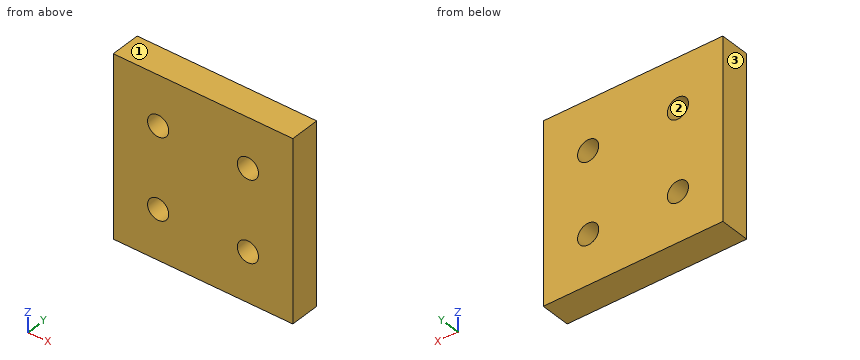
Autodesk Inventor part; units mm, degrees
ref_plane "YZ Plane" through (0, 0, 0) normal (1, 0, 0) x (0, 1, 0)
ref_plane "XZ Plane" through (0, 0, 0) normal (0, 1, 0) x (-1, 0, 0)
ref_plane "XY Plane" through (0, 0, 0) normal (0, 0, 1) x (1, 0, 0)
sketch "Sketch1" plane through (0, 0, 0) normal (0, 1, 0) x (-1, 0, 0)
  line L0 (-19.05, 19.05) -> (19.05, 19.05)
  line L1 (19.05, 19.05) -> (19.05, -19.05)
  line L2 (19.05, -19.05) -> (-19.05, -19.05)
  line L3 (-19.05, -19.05) -> (-19.05, 19.05)
  line L4 (-19.05, 19.05) -> (19.05, -19.05) construction
  line L5 (19.05, 19.05) -> (-19.05, -19.05) construction
  point P0 (0, 0)
  dimension "d0" = 38.1
  dimension "d1" = 38.1
extrude "Extrusion1" add sketch "Sketch1" along normal blind 6.35
sketch "Sketch2" plane through (0, 6.35, 0) normal (0, 1, 0) x (1, 0, 0)
  line L0 (-19.05, -19.05) -> (19.05, -19.05) construction
  line L1 (19.05, -19.05) -> (19.05, 19.05) construction
  line L2 (19.05, 19.05) -> (-19.05, 19.05) construction
  line L3 (-19.05, 19.05) -> (-19.05, -19.05) construction
  point P0 (0, 0)
  point P1 (-9.525, -8.5725)
  point P2 (-9.525, 8.5725)
  point P3 (9.525, -8.5725)
  point P4 (9.525, 8.5725)
  dimension "d6" = 17.145
  dimension "d9" = 19.05
  dimension "d12" = 8.5725
  dimension "d13" = 9.525
hole "Hole1" at (-9.525, 6.35, 8.5725) at (-9.525, 6.35, -8.5725) at (9.525, 6.35, 8.5725) at (9.525, 6.35, -8.5725) direction (0, -1, 0) diameter 4.4958 end through all
properties part number "holestandard" material "Aluminum 6061"
Part model, mm, in its own coordinate system. Face numbers are marked on the shaded views. Coordinates: 2 decimals unless noted, no trailing zeros. Order: outer loops, then holes, each group sorted by start corner. A loop starts at its lowest first (then second) coordinate and runs counter-clockwise, first axis right, second up. Notation, with made-up numbers: M 80.5,0 L 119.5,0 A17 cw 119.5,15 Z; hole C 70,-34 d3. An arc over 180 degrees is marked long. Use a Markdown table: item, result.
(1) Flat gauge pin, fed straight in: pin 1 (7 mm diameter, centred on x = 9.52, z = 8.57, fed in from +Y). Where does the tip first touch, or does it go through?
A:
| item | result |
|---|---|
| pin 1 | stops at y = 6.35 |
(2) Cut at A-A on z = 7. Write the cut outline in (x, y), then the cut area to 3 significant figures.
A:
| item | result |
|---|---|
| outline | M -19.05,0 L -11.13,0 L -11.13,6.35 L -19.05,6.35 Z; M -7.92,0 L 7.92,0 L 7.92,6.35 L -7.92,6.35 Z; M 11.13,0 L 19.05,0 L 19.05,6.35 L 11.13,6.35 Z |
| area | 201 mm^2 |
(3) Pull direction X, two halves, no side cores. Call the marked faces 1, 2 and 3: released by +X, released by -X, zero draft, split by the parting line, or undercut.
A:
| item | result |
|---|---|
| face 1 | zero draft |
| face 2 | undercut |
| face 3 | released by -X |
(4) Cut at C-C on y = 4. State how many separate pieces and enclosed holes the cut face has, then the cut area to 3 significant figures.
A:
| item | result |
|---|---|
| separate pieces | 1 |
| enclosed holes | 4 |
| area | 1,390 mm^2 |
(5) Cut at B-B on x = 10.5. Write the cut outline in (y, z).
A:
| item | result |
|---|---|
| outline | M 0,-19.05 L 6.35,-19.05 L 6.35,-10.6 L 0,-10.6 Z; M 0,-6.55 L 6.35,-6.55 L 6.35,6.55 L 0,6.55 Z; M 0,10.6 L 6.35,10.6 L 6.35,19.05 L 0,19.05 Z |
(6) Probe L1, parallel to X at y = 5.25, z = 7.5; L2, parallel to X at y = 2.75, z = 9; L3, parallel to Z at x = 8.5, y = 0.75. List the from-to ranges inside material, lowest first.
A:
| item | result |
|---|---|
| L1 | x = -19.05 to -11.5, -7.55 to 7.55, 11.5 to 19.05 |
| L2 | x = -19.05 to -11.73, -7.32 to 7.32, 11.73 to 19.05 |
| L3 | z = -19.05 to -10.57, -6.57 to 6.57, 10.57 to 19.05 |
